Build history of the part. All positions in model axes, mm. A direction names the side the tool comes from. Round coordinates to 2 decimals unless told otherwise and drop trailing zeros. Loops run counter-clockwise (first coordinate to the right, second up) from the corner with the lowest first, then second, coordinate; pieces in that order, holes last. Notation, with made-up numbers: (47, 44.5) - (87, 44.5) arc R26 ccw to (87, 80.5) - close; hole circle Ø2 at (-18, 0). An arc over 180 degrees is marked (long way). Use one line per item in the form item = value. Start each with the question number.
Q1. 3-axis set-ups, long thin cutter, end or side, ignore diameter. For faces 3 (the face through (6, -49.2, 6)), 4 (the face through (5, 5, -16.75)), 5 (the face through (-3, -30, -10.85)): which of +Z, -Z, +X, -X, +Y, -Y reach the whole face in a straight line?
Q2. Pin check, flat tips, straight feed: pin 1 (11 mm diameter, centred on y = -30.5, z = -4.5, fed in from -X); pin 2 (6 mm diameter, centred on x = 21, z = -45, fed in from -Y); pin 3 (10 mm diameter, centred on x = -12, y = -44, fed in from +Z); pin 4 (21 mm diameter, centred on x = -1.5, z = -8.5, fed in from -Y). Stop position of each tip, or through.
Q3. Mould opens along Z. For faces 1 (the face through (-12.93, 1.972, 16.863)), 2 (the face through (7, -65, -7)) say: released by +Z, released by -Z, zero draft, split by the parting line, or undercut.
Q4. Saw through at B-B (x = 0). Give the cut face in (y, z).
Q5. Drill centre lines: line 1 (X direction, y = 1, z = 0); line 2 (Z direction, x = -9, y = -44); line 3 (Z direction, x = 5, y = 4.5). Where is each one in solid material? Low to high.
Q6. Saw through at C-C (z = 0). Give the cut face in (x, y), then the cut area to 3 significant figures.
Q7. Saw through at A-A (y = -41). Give the cut face in (x, z).
Q8. Saw through at D-D (y = -2). Give the cut face in (x, z).
```python
from build123d import *

# Parameters (mm, degrees)
BOSS_EXTRUDE1_DEPTH = 6.8
SKETCH2_R           = 12.5
SKETCH2_R_2         = 9
BOSS_EXTRUDE2_DEPTH = 2
SKETCH3_W           = 4.7
SKETCH3_H           = 3.2
CUT_EXTRUDE1_DEPTH  = 10
SKETCH7_R           = 21.25
CUT_EXTRUDE4_DEPTH  = 4
SKETCH8_W           = 21.7
SKETCH8_H           = 21.7
BOSS_EXTRUDE3_DEPTH = 69
SKETCH9_W           = 16.5
SKETCH9_H           = 16.5
CUT_EXTRUDE5_DEPTH  = 56
SKETCH10_R          = 6
CUT_EXTRUDE6_DEPTH  = 99
CUT_EXTRUDE7_DEPTH  = 38


with BuildPart() as part:
    # Sketch1 → Boss-Extrude1 (new body)
    with BuildSketch(Plane(origin=(0, 0, 0), x_dir=(1, 0, 0), z_dir=(0, 1, 0))):
        with BuildLine():
            Line((-12.289695868, 83.033281734), (-26.791536992, 4.97755418))
            ThreePointArc((-26.791536992, 4.97755418), (0, -27.25), (26.791536992, 4.97755418))
            Line((26.791536992, 4.97755418), (12.289695868, 83.033281734))
            ThreePointArc((12.289695868, 83.033281734), (0, 93.25), (-12.289695868, 83.033281734))
        make_face()
    extrude(amount=BOSS_EXTRUDE1_DEPTH)

    # Sketch2 → Boss-Extrude2 (add)
    with BuildSketch(Plane(origin=(0, 6.8, 0), x_dir=(1, 0, 0), z_dir=(0, 1, 0))):
        with Locations(Location((0, 80.75, 0), (0, 0, 169.47511628))):
            Circle(SKETCH2_R)
        with Locations(Location((0, 80.75, 0), (0, 0, 270))):
            Circle(SKETCH2_R_2, mode=Mode.SUBTRACT)
    extrude(amount=BOSS_EXTRUDE2_DEPTH)

    # Sketch3 → Cut-Extrude1 (cut)
    with BuildSketch(Plane(origin=(0, 6.8, 0), x_dir=(1, 0, 0), z_dir=(0, 1, 0))):
        with Locations((4.65, 18.35)):
            Rectangle(SKETCH3_W, SKETCH3_H)
        with Locations((-4.65, 18.35)):
            Rectangle(SKETCH3_W, SKETCH3_H)
    extrude(amount=-CUT_EXTRUDE1_DEPTH, mode=Mode.SUBTRACT)

    # Sketch7 → Cut-Extrude4 (cut)
    with BuildSketch(Plane.XZ):
        with Locations(Location((0, 0, 0), (0, 0, 270))):
            Circle(SKETCH7_R)
    extrude(amount=-CUT_EXTRUDE4_DEPTH, mode=Mode.SUBTRACT)

    # Sketch8 → Boss-Extrude3 (add)
    with BuildSketch(Plane.XZ.offset(-4)):
        Rectangle(SKETCH8_W, SKETCH8_H)
    extrude(amount=BOSS_EXTRUDE3_DEPTH)

    # Sketch9 → Cut-Extrude5 (cut)
    with BuildSketch(Plane(origin=(0, 6.8, 0), x_dir=(1, 0, 0), z_dir=(0, 1, 0))):
        Rectangle(SKETCH9_W, SKETCH9_H)
    extrude(amount=-CUT_EXTRUDE5_DEPTH, mode=Mode.SUBTRACT)

    # Sketch10 → Cut-Extrude6 (cut)
    with BuildSketch(Plane.XZ.offset(65)):
        with Locations(Location((0, 0, 0), (0, 0, 270))):
            Circle(SKETCH10_R)
    extrude(amount=-CUT_EXTRUDE6_DEPTH, mode=Mode.SUBTRACT)

    # Sketch11 → Cut-Extrude7 (cut)
    with BuildSketch(Plane.XZ.offset(65)):
        with BuildLine():
            Line((-6, 2.5), (-5.454356057, 2.5))
            ThreePointArc((-5.454356057, 2.5), (-6, 0), (-5.454356057, -2.5))
            Line((-5.454356057, -2.5), (-6, -2.5))
            Line((-6, -2.5), (-10.85, -2.5))
            Line((-10.85, -2.5), (-10.85, 2.5))
            Line((-10.85, 2.5), (-6, 2.5))
        make_face()
        with BuildLine():
            Line((-2.5, 6), (-2.5, 5.454356057))
            ThreePointArc((-2.5, 5.454356057), (0, 6), (2.5, 5.454356057))
            Line((2.5, 5.454356057), (2.5, 6))
            Line((2.5, 6), (2.5, 10.85))
            Line((2.5, 10.85), (-2.5, 10.85))
            Line((-2.5, 10.85), (-2.5, 6))
        make_face()
        with BuildLine():
            Line((-2.5, -6), (-2.5, -10.85))
            Line((-2.5, -10.85), (2.5, -10.85))
            Line((2.5, -10.85), (2.5, -6))
            Line((2.5, -6), (2.5, -5.454356057))
            ThreePointArc((2.5, -5.454356057), (0, -6), (-2.5, -5.454356057))
            Line((-2.5, -5.454356057), (-2.5, -6))
        make_face()
        with BuildLine():
            Line((6, -2.5), (10.85, -2.5))
            Line((10.85, -2.5), (10.85, 2.5))
            Line((10.85, 2.5), (6, 2.5))
            Line((6, 2.5), (5.454356057, 2.5))
            ThreePointArc((5.454356057, 2.5), (6, 0), (5.454356057, -2.5))
            Line((5.454356057, -2.5), (6, -2.5))
        make_face()
    extrude(amount=-CUT_EXTRUDE7_DEPTH, mode=Mode.SUBTRACT)


solid = part.part
```
Report:
q1.face_3 = +Y
q1.face_4 = +Y, -Y
q1.face_5 = -Y
q2.pin_1 = -10.85
q2.pin_2 = 0
q2.pin_3 = 10.85
q2.pin_4 = -65
q3.face_1 = undercut
q3.face_2 = zero draft
q4.outline = (-27, -10.85) - (4, -10.85) - (4, -21.25) - (0, -21.25) - (0, -93.25) - (8.8, -93.25) - (8.8, -89.75) - (6.8, -89.75) - (6.8, -71.75) - (8.8, -71.75) - (8.8, -68.25) - (6.8, -68.25) - (6.8, -8.25) - (-27, -8.25) - close; (-27, 8.25) - (6.8, 8.25) - (6.8, 27.25) - (0, 27.25) - (0, 21.25) - (4, 21.25) - (4, 10.85) - (-27, 10.85) - close
q5.line_1 = -27.25 to -21.25, -10.85 to -8.25, 8.25 to 10.85, 21.25 to 27.25
q5.line_2 = -10.85 to -2.5, 2.5 to 10.85
q5.line_3 = -92.21 to -19.95, -16.75 to -8.25, 8.25 to 26.79
q6.outline = (-27.25, 0) - (-21.25, 0) - (-21.25, 4) - (-10.85, 4) - (-10.85, -27) - (-8.25, -27) - (-8.25, 6.8) - (-27.25, 6.8) - close; (8.25, -27) - (10.85, -27) - (10.85, 4) - (21.25, 4) - (21.25, 0) - (27.25, 0) - (27.25, 6.8) - (8.25, 6.8) - close
q6.area = 316 mm²
q7.outline = (-10.85, -10.85) - (-2.5, -10.85) - (-2.5, -8.25) - (-8.25, -8.25) - (-8.25, -2.5) - (-10.85, -2.5) - close; (-10.85, 2.5) - (-8.25, 2.5) - (-8.25, 8.25) - (-2.5, 8.25) - (-2.5, 10.85) - (-10.85, 10.85) - close; (2.5, -10.85) - (10.85, -10.85) - (10.85, -2.5) - (8.25, -2.5) - (8.25, -8.25) - (2.5, -8.25) - close; (2.5, 8.25) - (8.25, 8.25) - (8.25, 2.5) - (10.85, 2.5) - (10.85, 10.85) - (2.5, 10.85) - close
q8.outline = (-10.85, -10.85) - (10.85, -10.85) - (10.85, 10.85) - (-10.85, 10.85) - close; hole (-8.25, -8.25) - (8.25, -8.25) - (8.25, 8.25) - (-8.25, 8.25) - close
